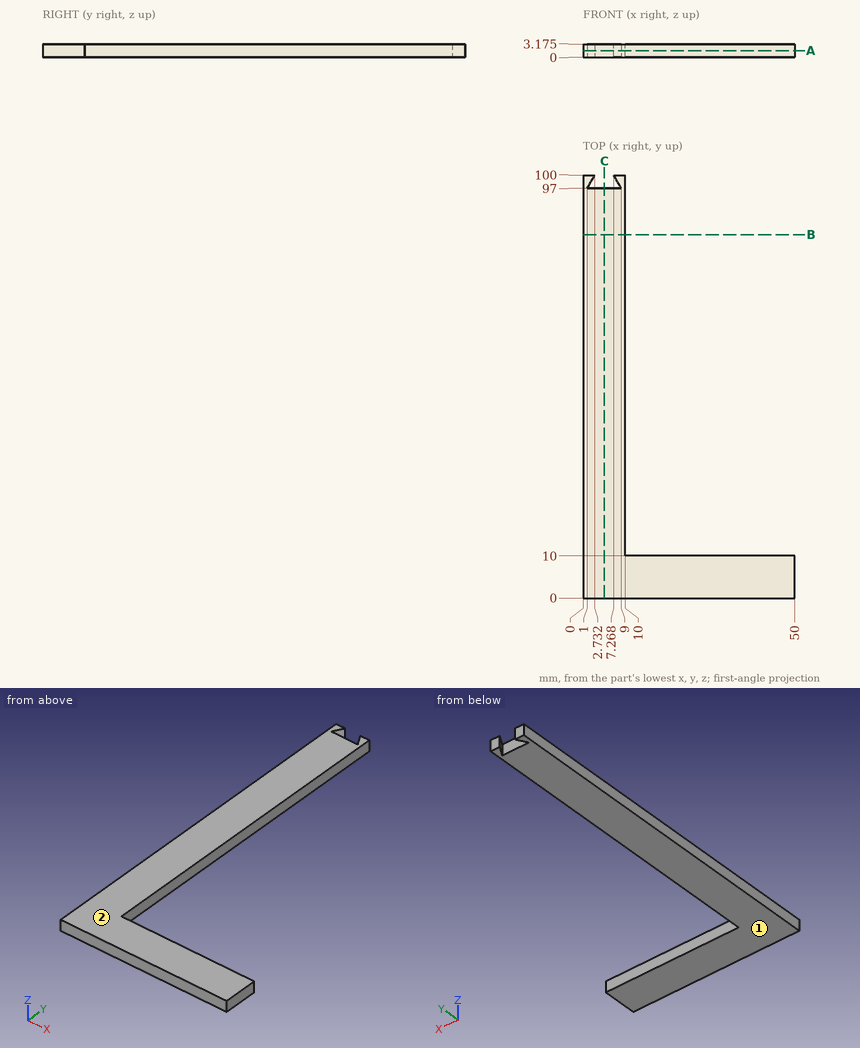
Print and shaded views of the part. All mm, measured from the part's lowest x, y and z. Round coordinates to 2 decimals unless told otherwise and drop trailing zeros. Write each loop counter-clockwise with the first axis right and the second up, starting at its lowest first coordinate (ties: lowest second). Pieces come first, ordered by that corner, then holes.
Item 1: Two-plate mould, pull along Z, no slides. Class the marked faces 1 and 2: +Z half, -Z half, draft (parallel to the pull), parting line (faces both ways), or undercut.
Results:
face 1: -Z half
face 2: +Z half
Item 2: Probe L1, parallel to Y at x = 28.5, z = 2.15; L2, parallel to Y at x = 4.5, z = 0.2. List the from-to ranges inside material, lowest first.
Results:
L1: y = 0 to 10
L2: y = 0 to 97
Item 3: Cut at A-A, the plane z = 1.6. Give the cut face in (x, y).
Results:
outline: (0, 0) - (50, 0) - (50, 10) - (10, 10) - (10, 100) - (7.27, 100) - (9, 97) - (1, 97) - (2.73, 100) - (0, 100) - close
Item 4: Drop flat-ended pins along their axis: pin 1 Ø1.6 at (x, z) = (26.5, 1) entering from +Y; pin 2 Ø3 at (x, y) = (8, 80) entering from -Z; pin 3 Ø1.6 at (y, z) = (66, 1) entering from +X. Give the stop position or say it passes through.
Results:
pin 1: stops at y = 10
pin 2: stops at z = 0
pin 3: stops at x = 10
Item 5: Cut at B-B, the plane y = 86. Give the cut face in (x, z) (3 decimals).
Results:
outline: (0, 0) - (10, 0) - (10, 3.175) - (0, 3.175) - close
Item 6: Cut at C-C, the plane x = 5. Give the cut face in (y, z) (3 decimals).
Results:
outline: (0, 0) - (97, 0) - (97, 3.175) - (0, 3.175) - close
